```python
from build123d import *

# Parameters (mm, degrees)
F2_DEPTH = 9.525
F3_R     = 3.81
F4_R     = 1.524


with BuildPart() as f2:
    # F1 (on Top) → F2 (new body, symmetric)
    with BuildSketch(Plane.XY):
        Polygon((10.287, 10.287), (10.287, -10.287), (6.477, -10.287), (6.477, -12.573), (12.573, -12.573), (12.573, 12.573), (-12.573, 12.573), (-12.573, -12.573), (-7.800612, -12.573), (-4.440114, -18.427097), (-2.457546, -17.28902), (-6.477, -10.287), (-10.287, -10.287), (-10.287, 10.287), align=None)
    extrude(amount=F2_DEPTH, both=True)

    # F3
    f3_edges = [f2.edges().sort_by_distance(p)[0] for p in [
        (-6.477, -10.287, 0),
    ]]
    fillet(f3_edges, radius=F3_R)

    # F4
    f4_edges = [f2.edges().sort_by_distance(p)[0] for p in [
        (-7.800612, -12.573, 0),
    ]]
    fillet(f4_edges, radius=F4_R)


solid = f2.part
```
Verification items for the finished model (mm, model axes). A direction names the side the tool comes from. Give positions to 0.01 mm unless a question says otherwise; leave off trailing zeros. Loops run counter-clockwise (first coordinate to the right, second up) from the corner with the lowest first, then second, coordinate; pieces in that order, holes last.
1. Section check A-A, the plane y = -3. Enter the section's corners in (x, z) (3 decimals).
2. Thickness scan on line 1 (X direction, y = 6.5, z = 4.5); line 2 (Y direction, x = -11, z = -8.5). Record the ranges inside material, lowest first.
3. Section check C-C, the plane z = 8.75. Enter the section's corners in (x, y), then the cut area to 3 significant figures.
4. Section check D-D, the plane x = 0.25. Enter the section's corners in (y, z) (3 decimals), then the cut area to 3 significant figures.
5. Section check B-B, the plane x = -4. Enter the section's corners in (y, z) (3 decimals), then the cut area to 3 significant figures.
6. Go/stop test with flat-tipped pins: pin 1 Ø1.5 at (x, z) = (1, 5.5) entering from -Y; pin 2 Ø1.2 at (x, z) = (-11.5, 3) entering from -Y. Record where each tip stops, or that it passes through.
7. Mould release check, pull along Y, two halves, no side actions. Record for faces 6 (the flat face through (6.477, -11, 0)), 7 (the flat face through (-5.92, -15.85, 0.13)), 8 (the flat face through (-10.287, 0, 0)), 9 (the flat face through (10.287, 0, 0)): released by +Y, released by -Y, zero draft, split by the parting line, or undercut.
8. Set-up check for faces 1 (the flat face through (-9, -10.287, 0)), 2 (the flat face through (-11, -12.573, 0)), 3 (the flat face through (9, -12.573, 0)), 4 (the flat face through (12.573, 0, 0)), 5 (the flat face through (0, 12.573, 0)): record each of +Z, -Z, +X, -X, +Y, -Y from which the full face is reachable in a straight line by a thin tool's end or side.
Geometry says:
1. outline: (-12.573, -9.525) - (-10.287, -9.525) - (-10.287, 9.525) - (-12.573, 9.525) - close; (10.287, -9.525) - (12.573, -9.525) - (12.573, 9.525) - (10.287, 9.525) - close
2. line 1: x = -12.57 to -10.29, 10.29 to 12.57
2. line 2: y = -12.57 to 12.57
3. outline: (-12.57, -12.57) - (-8.68, -12.57) arc R1.52 cw to (-7.36, -13.34) - (-4.44, -18.43) - (-2.46, -17.29) - (-5.38, -12.2) arc R3.81 ccw to (-8.68, -10.29) - (-10.29, -10.29) - (-10.29, 10.29) - (10.29, 10.29) - (10.29, -10.29) - (6.48, -10.29) - (6.48, -12.57) - (12.57, -12.57) - (12.57, 12.57) - (-12.57, 12.57) - close
3. area: 194 mm2
4. outline: (10.287, -9.525) - (12.573, -9.525) - (12.573, 9.525) - (10.287, 9.525) - close
4. area: 43.5 mm2
5. outline: (-18.174, -9.525) - (-14.602, -9.525) - (-14.602, 9.525) - (-18.174, 9.525) - close; (10.287, -9.525) - (12.573, -9.525) - (12.573, 9.525) - (10.287, 9.525) - close
5. area: 112 mm2
6. pin 1: stops at y = 10.29
6. pin 2: stops at y = -12.57
7. face 6: zero draft
7. face 7: released by -Y
7. face 8: undercut
7. face 9: undercut
8. face 1: +Z, -Z
8. face 2: +Z, -Z, -X, -Y
8. face 3: +Z, -Z, +X, -Y
8. face 4: +Z, -Z, +X, +Y, -Y
8. face 5: +Z, -Z, +X, -X, +Y
